Job drawing, mm, ordinate dimensions from the low corner. One solid piece. A direction names the side the tool comes from. Coordinates: 2 decimals unless noted, no trailing zeros. Loops run counter-clockwise (first coordinate to the right, second up) from the corner with the lowest first, then second, coordinate; pieces in that order, holes last. Notation, with made-up numbers: M -6,13.25 L 31,13.25 A15 ccw 31,31.25 Z; hole C 35.5,-10 d11. An arc over 180 degrees is marked long. Answer as a JSON object with one key per item and string values. Group by question number.
1. Saw through at A-A on x = 2.5. Write the cut outline in (y, z).
2. 3-axis set-ups, long thin cutter, end or side, ignore diameter. For the marked faces 1, 2 and 3: which of +Z, -Z, +X, -X, +Y, -Y reach the whole face in a straight line?
3. Saw through at B-B on z = 29.5. Write the cut outline in (x, y).
4. Drop flat-ended pins along their axis: pin 1 Ø8 at (x, z) = (17.5, 16.5) entering from -Y; pin 2 Ø2.5 at (x, z) = (2.5, 29.5) entering from -Y; pin 3 Ø1.5 at (x, y) = (9, 6) entering from +Z; pin 4 Ø1.5 at (x, y) = (21.5, 7.5) entering from +Z. Give the stop position or say it passes through.
5. Drill centre lines: L1, parallel to X at y = 16.2, z = 29.5; L2, parallel to X at y = 10.75, z = 13.5; L3, parallel to Y at x = 8.5, z = 11. Where is each one in solid material? Low to high.
6. Saw through at D-D on z = 20. Write the cut outline in (x, y).
7. Saw through at C-C on y = 11. Write the cut outline in (x, z).
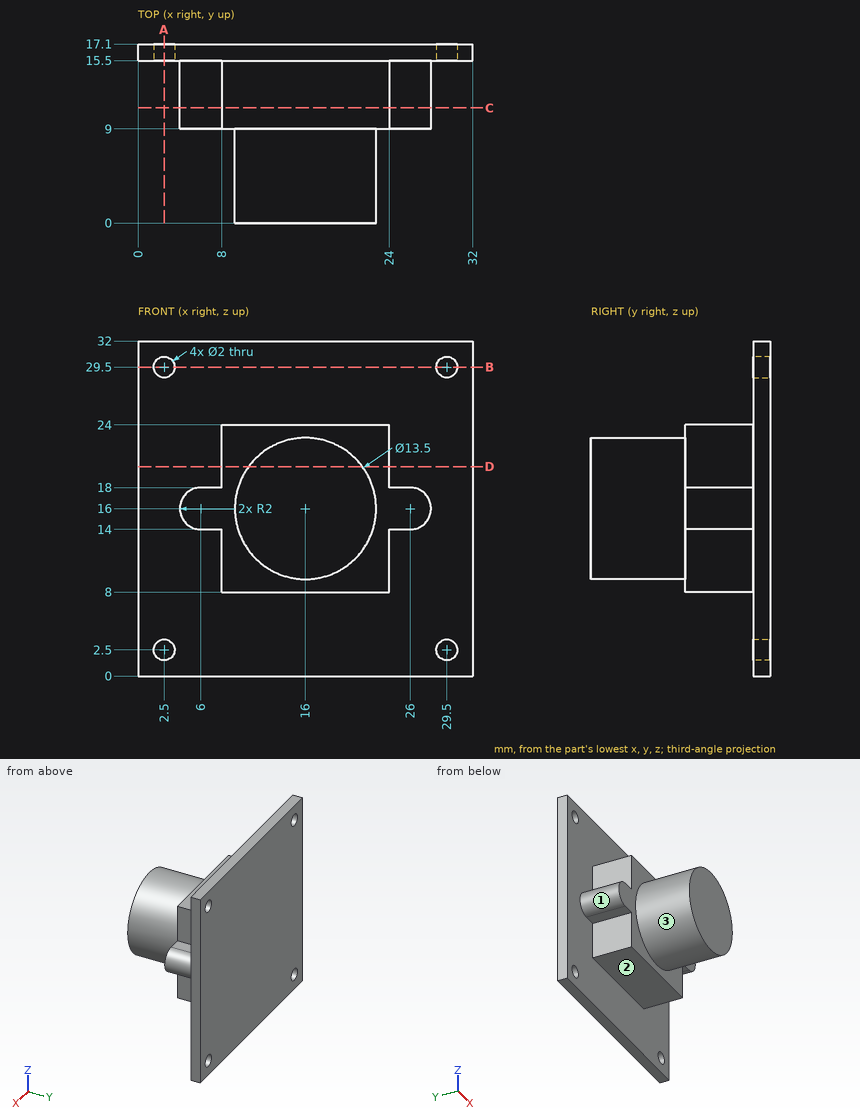
Outcome:
{
 "1": {"outline": "M 15.5,0 L 17.1,0 L 17.1,1.5 L 15.5,1.5 Z; M 15.5,3.5 L 17.1,3.5 L 17.1,28.5 L 15.5,28.5 Z; M 15.5,30.5 L 17.1,30.5 L 17.1,32 L 15.5,32 Z"},
 "2": {"face 1": "-X, -Y", "face 2": "-Z, +X, -X, -Y", "face 3": "-Y"},
 "3": {"outline": "M 0,15.5 L 1.5,15.5 L 1.5,17.1 L 0,17.1 Z; M 3.5,15.5 L 28.5,15.5 L 28.5,17.1 L 3.5,17.1 Z; M 30.5,15.5 L 32,15.5 L 32,17.1 L 30.5,17.1 Z"},
 "4": {"pin 1": "stops at y = 0", "pin 2": "stops at y = 15.5", "pin 3": "stops at z = 18.55", "pin 4": "stops at z = 20.8"},
 "5": {"L1": "x = 0 to 1.5, 3.5 to 28.5, 30.5 to 32", "L2": "x = 8 to 24", "L3": "y = 9 to 17.1"},
 "6": {"outline": "M 0,15.5 L 8,15.5 L 8,9 L 10.56,9 L 10.56,0 L 21.44,0 L 21.44,9 L 24,9 L 24,15.5 L 32,15.5 L 32,17.1 L 0,17.1 Z"},
 "7": {"outline": "M 6,14 L 8,14 L 8,8 L 24,8 L 24,14 L 26,14 A2 ccw 26,18 L 24,18 L 24,24 L 8,24 L 8,18 L 6,18 A2 ccw Z"}
}
